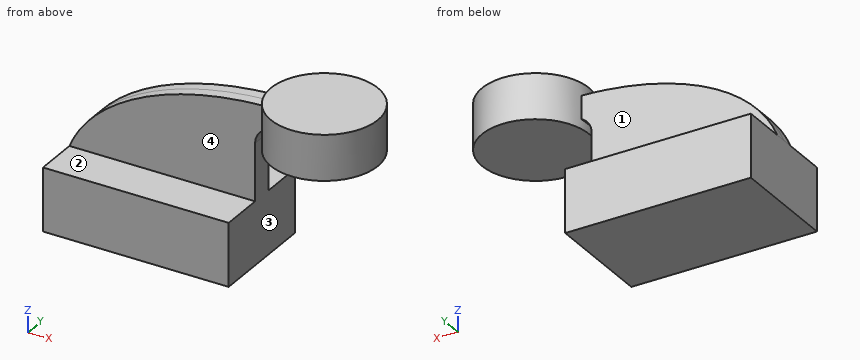
from build123d import *

# Parameters (mm, degrees)
F1_DEPTH = 25
F2_DEPTH = 5


with BuildPart() as f1:
    # F0 (on Front) → F1 (new body, symmetric)
    with BuildSketch(Plane.XZ):
        Polygon((32.5, 14.412519), (-42.5, 14.412519), (-42.5, -14.412519), (42.5, -14.412519), (42.5, 14.412519), align=None)
    extrude(amount=F1_DEPTH, both=True)

    # F0 (on Front) → F2 (join, symmetric)
    with BuildSketch(Plane.XZ):
        with BuildLine():
            Line((32.5, 40.587481), (32.5, 14.412519))
            Line((32.5, 14.412519), (42.5, 14.412519))
            Line((42.5, 14.412519), (42.5, 40.587481))
            ThreePointArc((42.5, 40.587481), (44.843146, 46.244336), (50.5, 48.587481))
            Line((50.5, 48.587481), (65.721087, 48.587481))
            Line((65.721087, 48.587481), (65.721087, 58.587481))
            Line((65.721087, 58.587481), (50.5, 58.587481))
            add(Edge.make_bspline(
                [(50.123601, 58.583546), (50.249035, 58.584995), (50.374501, 58.586307), (50.5, 58.587481)],
                knots=[102.657738, 102.657738, 102.657738, 102.657738, 102.958377, 102.958377, 102.958377, 102.958377], degree=3))
            ThreePointArc((50.123601, 58.583546), (37.639689, 53.181623), (32.5, 40.587481))
        make_face()
        with BuildLine():
            add(Edge.make_bspline(
                [(-42.5, 14.412519), (-31.693433, 41.543898), (7.292415, 58.088539), (50.123601, 58.583546)],
                knots=[0, 0, 0, 0, 102.657738, 102.657738, 102.657738, 102.657738], degree=3))
            Line((-42.5, 14.412519), (32.5, 14.412519))
            Line((32.5, 14.412519), (32.5, 40.587481))
            ThreePointArc((32.5, 40.587481), (37.639689, 53.181623), (50.123601, 58.583546))
        make_face()
    extrude(amount=F2_DEPTH, both=True)

    # F0 (on Front) → F3 (revolve)
    with BuildSketch(Plane.XZ):
        Polygon((71.16668, 64.222187), (71.16668, 58.587481), (71.16668, 48.587481), (71.16668, 43.468155), (95.699124, 43.468155), (95.699124, 64.222187), align=None)
    revolve(axis=Axis((71.16668, 0, 53.845171), (0, 0, 1)))


solid = f1.part
For this review, take the finished solid that the model builds, in its own axes (mm). Face numbers are marked on the shaded views. A direction names the side the tool comes from. Give positions to 0.01 mm unless a question says otherwise; leave off trailing zeros. Loops run counter-clockwise (first coordinate to the right, second up) from the corner with the lowest first, then second, coordinate; pieces in that order, holes last. Notation, with made-up numbers: M 82.5,27 L 116.5,27 A13 ccw 116.5,33 Z; hole C 76,5.25 d7. An arc over 180 degrees is marked long. Answer as a JSON object with one key per item and string values. Group by question number.
Q1. Insertion check: P1, Ø3, axis at x = -3.5, y = -17.5, coming from the +Z side; P2, Ø8, axis at x = 73, y = 5, coming from the -Z side; P3, Ø10, axis at x = 50, z = -5, coming from the +Y side. Each pin has a flat end and moves straight along its axis. Give the tip position at first contact, or say it passes through.
Q2. Add section D-D on x = 58.5. Give the boundary of the cut face in (y, z).
Q3. Add section B-B on z = 6. Give the boundary of the cut face in (x, y).
Q4. Tool access review of the marked faces 1, 2, 3 and 4: name each direction out of +Z, -Z, +X, -X, +Y, -Y from which nothing blocks a thin tool from reaching the whole face with its end or side.
Q5. For probe 1 along Z at (x, y) = (-21, 8.5); probe 2 along Y at (x, z) = (8, 20.5); probe 3 along X at (y, z) = (11, -1.5), list the stretches that pass through material, from the lowest coordinate up. Write a range as [from, to].
Q6. Add section A-A on y = -15. Give the boundary of the cut face in (x, z).
Q7. Add section C-C on y = 12. Give the boundary of the cut face in (x, z).
Checked values:
{
 "1": {"P1": "z = 14.41", "P2": "z = 43.47", "P3": "through"},
 "2": {"outline": "M -21.01,43.47 L 21.01,43.47 L 21.01,64.22 L -21.01,64.22 Z"},
 "3": {"outline": "M -42.5,-25 L 42.5,-25 L 42.5,25 L -42.5,25 Z"},
 "4": {"face 1": "+Z, -X, +Y", "face 2": "+Z, +X, -X, -Y", "face 3": "-Z, +X, +Y, -Y", "face 4": "+Z, -X, -Y"},
 "5": {"probe 1": "[-14.41, 14.41]", "probe 2": "[-5, 5]", "probe 3": "[-42.5, 42.5]"},
 "6": {"outline": "M -42.5,-14.41 L 42.5,-14.41 L 42.5,14.41 L -42.5,14.41 Z; M 51.75,43.47 L 90.58,43.47 L 90.58,64.22 L 51.75,64.22 Z"},
 "7": {"outline": "M -42.5,-14.41 L 42.5,-14.41 L 42.5,14.41 L -42.5,14.41 Z; M 49.77,43.47 L 92.56,43.47 L 92.56,64.22 L 49.77,64.22 Z"}
}
